from build123d import *

# Parameters (mm, degrees)
SKETCH001_R   = 47.5
SKETCH001_R_2 = 3.5
PAD_DEPTH     = 6.35
SKETCH_R      = 3.4
HOLE_DEPTH    = 6.351


with BuildPart() as part:
    # Sketch001 → Pad (new body)
    with BuildSketch(Plane.XY):
        Circle(SKETCH001_R)
        Circle(SKETCH001_R_2, mode=Mode.SUBTRACT)
        with BuildLine():
            ThreePointArc((8.214313, 12.491428), (0, 14.950275), (-8.214313, 12.491428))
            ThreePointArc((-11.785687, 17.922384), (-12.715478, 13.421219), (-8.214313, 12.491428))
            ThreePointArc((11.785687, 17.922384), (0, 21.450275), (-11.785687, 17.922384))
            ThreePointArc((8.214313, 12.491428), (12.715478, 13.421219), (11.785687, 17.922384))
        make_face(mode=Mode.SUBTRACT)
        with BuildLine():
            ThreePointArc((-8.214313, -12.491428), (0, -14.950275), (8.214313, -12.491428))
            ThreePointArc((11.785687, -17.922384), (12.715478, -13.421219), (8.214313, -12.491428))
            ThreePointArc((-11.785687, -17.922384), (0, -21.450275), (11.785687, -17.922384))
            ThreePointArc((-8.214313, -12.491428), (-12.715478, -13.421219), (-11.785687, -17.922384))
        make_face(mode=Mode.SUBTRACT)
    extrude(amount=PAD_DEPTH)

    # Sketch → Hole (cut, through all)
    with BuildSketch(Plane.XY):
        with Locations((-35, 0)):
            Circle(SKETCH_R)
        with Locations((35, 0)):
            Circle(SKETCH_R)
    extrude(amount=HOLE_DEPTH, mode=Mode.SUBTRACT)


solid = part.part
CAD build for the part. Positions are in the model's coordinates, mm. A direction names the side the tool comes from. Give positions to 0.01 mm unless a question says otherwise; leave off trailing zeros. Loops run counter-clockwise (first coordinate to the right, second up) from the corner with the lowest first, then second, coordinate; pieces in that order, holes last. Notation, with made-up numbers: M -32.5,-2 L 19.5,-2 A28 ccw 19.5,21 Z; hole C -14,-21 d7. An arc over 180 degrees is marked long. Answer in a Markdown table with one row per item. Add a question column.
Item 1: Tool access for faces 4 (the face through (-0.12, -14.95, 3.13)), 5 (the face through (10, 1, 6.35)): list every direction of +Z, -Z, +X, -X, +Y, -Y with a clear straight run to the whole face (end or side of a thin tool).
Item 2: Band-saw the part on B-B on y = 0. Give the cut face in (x, z).
Item 3: Mould opens along X. For faces 1 (the face through (-10.3, -46.37, 3.13)), 2 (the face through (-0.17, -21.45, 3.13)), 3 (the face through (10, 1, 0)) say: +X half, -X half, draft (parallel to the pull), parting line (faces both ways), or undercut.
Item 4: Drop flat-ended pins along their axis: P1, Ø5.5, axis at x = 0, y = 0, coming from the +Z side; P2, Ø1, axis at x = -36.5, z = 0.5, coming from the +Y side; P3, Ø2, axis at x = 28, z = 2.5, coming from the +Y side; P4, Ø3, axis at y = 12.5, z = 2, coming from the -X side. Give the stop position or say it passes through.
Item 5: Band-saw the part on A-A on x = 0. Give the cut face in (y, z), then the cut area to 3 significant figures.
Item 6: Band-saw the part on D-D on x = -34. Give the cut face in (y, z), then the cut area to 3 significant figures.
Item 7: Band-saw the part on C-C on z = 5.25. Give the cut face in (x, y), then the cut area to 3 significant figures.
Item 8: Probe probe 1 along Y at (x, z) = (0, 1.5); probe 2 along Y at (x, z) = (35, 3.5); probe 3 along Y at (x, z) = (-9, 3.25). List the from-to ranges inside material, lowest first.
Reply:
| question | item | result |
|---|---|---|
| 1 | face 4 | +Z, -Z |
| 1 | face 5 | +Z, +X, -X, +Y, -Y |
| 2 | outline | M -47.5,0 L -38.4,0 L -38.4,6.35 L -47.5,6.35 Z; M -31.6,0 L -3.5,0 L -3.5,6.35 L -31.6,6.35 Z; M 3.5,0 L 31.6,0 L 31.6,6.35 L 3.5,6.35 Z; M 38.4,0 L 47.5,0 L 47.5,6.35 L 38.4,6.35 Z |
| 3 | face 1 | parting line |
| 3 | face 2 | undercut |
| 3 | face 3 | draft |
| 4 | P1 | passes through |
| 4 | P2 | stops at y = 30.99 |
| 4 | P3 | stops at y = 39.08 |
| 4 | P4 | stops at x = -46.21 |
| 5 | outline | M -47.5,0 L -21.45,0 L -21.45,6.35 L -47.5,6.35 Z; M -14.95,0 L -3.5,0 L -3.5,6.35 L -14.95,6.35 Z; M 3.5,0 L 14.95,0 L 14.95,6.35 L 3.5,6.35 Z; M 21.45,0 L 47.5,0 L 47.5,6.35 L 21.45,6.35 Z |
| 5 | area | 476 mm^2 |
| 6 | outline | M -33.17,0 L -3.25,0 L -3.25,6.35 L -33.17,6.35 Z; M 3.25,0 L 33.17,0 L 33.17,6.35 L 3.25,6.35 Z |
| 6 | area | 380 mm^2 |
| 7 | outline | C 0,0 d95; hole C -35,0 d6.8; hole M -11.79,-17.92 A21.45 ccw 11.79,-17.92 A3.25 ccw 8.21,-12.49 A14.95 cw -8.21,-12.49 A3.25 ccw Z; hole M -11.79,17.92 A3.25 ccw -8.21,12.49 A14.95 cw 8.21,12.49 A3.25 ccw 11.79,17.92 A21.45 ccw Z; hole C 0,0 d7; hole C 35,0 d6.8 |
| 7 | area | 6,640 mm^2 |
| 8 | probe 1 | y = -47.5 to -21.45, -14.95 to -3.5, 3.5 to 14.95, 21.45 to 47.5 |
| 8 | probe 2 | y = -32.11 to -3.4, 3.4 to 32.11 |
| 8 | probe 3 | y = -46.64 to -19.47, -12.11 to 12.11, 19.47 to 46.64 |
